```python
from build123d import *

# Parameters (mm, degrees)
BOSS_EXTRUDE1_DEPTH = 6
SKETCH2_W           = 7.6
SKETCH2_H           = 8.4
BOSS_EXTRUDE2_DEPTH = 4
SKETCH3_W           = 40
SKETCH3_H           = 30
BOSS_EXTRUDE3_DEPTH = 6
BOSS_EXTRUDE4_DEPTH = 2.5
BOSS_EXTRUDE5_DEPTH = 2.5
FILLET1_R           = 10
SKETCH8_R           = 1.6
CUT_EXTRUDE1_DEPTH  = 34.2
FILLET3_R           = 0.5
FILLET4_R           = 0.5
FILLET5_R           = 0.5
SKETCH9_R           = 14.329528823
CUT_EXTRUDE2_DEPTH  = 12.2
CUT_EXTRUDE3_DEPTH  = 3
FILLET6_R           = 0.5
FILLET7_R           = 1
FILLET8_R           = 1.5
FILLET9_R           = 0.3


with BuildPart() as part:
    # Sketch1 → Boss-Extrude1 (new body, symmetric)
    with BuildSketch(Plane(origin=(0, 0, 0), x_dir=(1, 0, 0), z_dir=(0, 1, 0))):
        Polygon((-8, 0), (8, 0), (8, 3.6), (4.3, 7.2), (-4.3, 7.2), (-8, 3.6), align=None)
    extrude(amount=BOSS_EXTRUDE1_DEPTH, both=True)

    # Sketch2 → Boss-Extrude2 (add)
    with BuildSketch(Plane(origin=(0, 0, -7.2), x_dir=(-1, 0, 0), z_dir=(0, 0, -1))):
        Rectangle(SKETCH2_W, SKETCH2_H)
    extrude(amount=BOSS_EXTRUDE2_DEPTH)

    # Sketch3 → Boss-Extrude3 (add)
    with BuildSketch(Plane(origin=(0, 0, -11.2), x_dir=(-1, 0, 0), z_dir=(0, 0, -1))):
        Rectangle(SKETCH3_W, SKETCH3_H)
    extrude(amount=BOSS_EXTRUDE3_DEPTH)

    # Sketch6 → Boss-Extrude4 (add, symmetric)
    with BuildSketch(Plane.ZY.offset(10)):
        Polygon((-29.2, 8), (-17.2, 8), (-17.2, 12), (-33.2, 12), (-33.2, -12), (-25.2, -12), (-25.2, -8), (-29.2, -8), align=None)
    extrude(amount=BOSS_EXTRUDE4_DEPTH, both=True)

    # Sketch7 → Boss-Extrude5 (add, symmetric)
    with BuildSketch(Plane(origin=(10, 0, 0), x_dir=(0, 0, -1), z_dir=(1, 0, 0))):
        Polygon((25.2, 12), (25.2, 8), (29.2, 8), (29.2, -8), (17.2, -8), (17.2, -12), (33.2, -12), (33.2, 12), align=None)
    extrude(amount=BOSS_EXTRUDE5_DEPTH, both=True)

    # Fillet1
    fillet1_edges = [part.edges().sort_by_distance(p)[0] for p in [
        (-20, -15, -14.2),
        (-20, 15, -14.2),
        (20, 15, -14.2),
        (20, -15, -14.2),
    ]]
    fillet(fillet1_edges, radius=FILLET1_R)

    # Sketch8 → Cut-Extrude1 (cut, through all)
    with BuildSketch(Plane.XY):
        Circle(SKETCH8_R)
    extrude(amount=-CUT_EXTRUDE1_DEPTH, mode=Mode.SUBTRACT)

    # Fillet3
    fillet3_edges = [part.edges().sort_by_distance(p)[0] for p in [
        (-6.15, 6, -5.4),
        (-8, 6, -1.8),
        (0, 6, 0),
        (8, 6, -1.8),
        (6.15, 6, -5.4),
        (8, -6, -1.8),
        (0, -6, 0),
        (-8, -6, -1.8),
        (-6.15, -6, -5.4),
        (0, -6, -7.2),
        (6.15, -6, -5.4),
        (0, 6, -7.2),
    ]]
    fillet(fillet3_edges, radius=FILLET3_R)

    # Fillet4
    fillet4_edges = [part.edges().sort_by_distance(p)[0] for p in [
        (-20, 0, -11.2),
        (-20, 0, -17.2),
        (0, -15, -11.2),
        (20, 0, -11.2),
        (0, 15, -11.2),
        (17.071067812, 12.071067812, -11.2),
        (17.071067812, -12.071067812, -11.2),
        (-17.071067812, 12.071067812, -11.2),
        (-17.071067812, -12.071067812, -11.2),
        (0, -15, -17.2),
        (0, 15, -17.2),
        (20, 0, -17.2),
        (17.071067812, 12.071067812, -17.2),
        (17.071067812, -12.071067812, -17.2),
        (-17.071067812, 12.071067812, -17.2),
        (-17.071067812, -12.071067812, -17.2),
    ]]
    fillet(fillet4_edges, radius=FILLET4_R)

    # Fillet5
    fillet5_edges = [part.edges().sort_by_distance(p)[0] for p in [
        (-3.8, 0, -11.2),
        (0, 4.2, -11.2),
        (3.8, 0, -11.2),
        (0, -4.2, -11.2),
    ]]
    fillet(fillet5_edges, radius=FILLET5_R)

    # Sketch9 → Cut-Extrude2 (cut, through all)
    with BuildSketch(Plane.XY.offset(-11.2)):
        Circle(SKETCH9_R)
    extrude(amount=CUT_EXTRUDE2_DEPTH, mode=Mode.SUBTRACT)

    # Sketch10 → Cut-Extrude3 (cut)
    with BuildSketch(Plane.XY.offset(-11.2)):
        Polygon((3.5, 0), (1.75, 3.031088913), (-1.75, 3.031088913), (-3.5, 0), (-1.75, -3.031088913), (1.75, -3.031088913), align=None)
    extrude(amount=-CUT_EXTRUDE3_DEPTH, mode=Mode.SUBTRACT)

    # Fillet6
    fillet6_edges = [part.edges().sort_by_distance(p)[0] for p in [
        (2.625, -1.515544457, -11.2),
        (2.625, 1.515544457, -11.2),
        (0, 3.031088913, -11.2),
        (-2.625, 1.515544457, -11.2),
        (-2.625, -1.515544457, -11.2),
        (0, -3.031088913, -11.2),
    ]]
    fillet(fillet6_edges, radius=FILLET6_R)

    # Fillet7
    fillet7_edges = [part.edges().sort_by_distance(p)[0] for p in [
        (-10, 8, -29.2),
        (-10, 12, -33.2),
        (-10, -12, -33.2),
        (-10, -12, -25.2),
        (-10, -8, -25.2),
        (-10, -8, -29.2),
        (10, -12, -33.2),
        (10, 12, -33.2),
        (10, 12, -25.2),
        (10, 8, -25.2),
        (10, 8, -29.2),
        (10, -8, -29.2),
    ]]
    fillet(fillet7_edges, radius=FILLET7_R)

    # Fillet8
    fillet8_edges = [part.edges().sort_by_distance(p)[0] for p in [
        (-7.5, 10, -17.2),
        (-10, 8, -17.2),
        (-10, 12, -17.2),
        (-12.5, 10, -17.2),
        (10, -12, -17.2),
        (7.5, -10, -17.2),
        (10, -8, -17.2),
        (12.5, -10, -17.2),
    ]]
    fillet(fillet8_edges, radius=FILLET8_R)

    # Fillet9
    fillet9_edges = [part.edges().sort_by_distance(p)[0] for p in [
        (-1.6, 0, -17.2),
    ]]
    fillet(fillet9_edges, radius=FILLET9_R)


solid = part.part
```
The listing builds one solid part. Answer for the finished solid, in the listing's coordinates (mm). A direction names the side the tool comes from. Coordinates: 2 decimals unless noted, no trailing zeros. Loops run counter-clockwise (first coordinate to the right, second up) from the corner with the lowest first, then second, coordinate; pieces in that order, holes last. Notation, with made-up numbers: M 37,-10 L 50,-10 A17 cw 50,18 Z; hole C 54.25,17.25 d11. An arc over 180 degrees is marked long. Answer as a JSON object with one key per item and string values. Group by question number.
Item 1: Each of these flat-tipped pins is pushed along its axis until it touches: P1, Ø2.5, axis at x = -10, z = -23.5, coming from the +Y side; P2, Ø11.5, axis at y = -2, z = -28.5, coming from the -X side; P3, Ø4, axis at x = 0, y = 0, coming from the +Z side. Where does it stop, or does it pass through?
Item 2: Which of the six approach directions +Z, -Z, +X, -X, +Y, -Y give full straight-line access (tool end or side, diameter ignored) to faces 1 (the face through (-10, -12, -29)), 2 (the face through (10.035, 8.301, -25.485)), 3 (the face through (-10.035, -11.715, -25.501)), 4 (the face through (10, -8, -24)), 5 (the face through (2.64, 1.49, -12.93))?
Item 3: Determine the mould class of faces 6 (the face through (-9.965, -8.301, -25.485)), 7 (the face through (-6.847, 10.049, -17.462)), 8 (the face through (7.5, 0, -31)) for opening direction X: +X half, -X half, draft (parallel to the pull), parting line (faces both ways), or undercut.
Item 4: Section A-A (z = -12.5) is taken. Write down the section's boundary in (x, y).
Item 5: Section D-D (z = -19.5) is taken. Write down the section's boundary in (x, y).
Item 6: Section C-C (z = -27.25) is taken. Write down the section's boundary in (x, y).
Item 7: Section B-B (x = 0) is taken. Write down the section's boundary in (y, z).
Item 8: Consider L1, parallel to Z at x = -11.5, y = -10; L2, parallel to Y at x = 0, z = -14.95; L3, parallel to X at y = 7, z = -31.5. Determine where each line is inside the solid, lowest interval first.
Solved:
{
 "1": {"P1": "stops at y = 12", "P2": "stops at x = -12.5", "P3": "stops at z = -14.2"},
 "2": {"face 1": "-Z, +X, -X, -Y", "face 2": "+X", "face 3": "-X, -Y", "face 4": "+X, -X", "face 5": "+Z"},
 "3": {"face 6": "draft", "face 7": "+X half", "face 8": "undercut"},
 "4": {"outline": "M -20,-5 A10 ccw -10,-15 L 10,-15 A10 ccw 20,-5 L 20,5 A10 ccw 10,15 L -10,15 A10 ccw -20,5 Z; hole M -3.5,0 L -1.75,-3.03 L 1.75,-3.03 L 3.5,0 L 1.75,3.03 L -1.75,3.03 Z"},
 "5": {"outline": "M -12.5,8 L -7.5,8 L -7.5,12 L -12.5,12 Z; M 7.5,-12 L 12.5,-12 L 12.5,-8 L 7.5,-8 Z"},
 "6": {"outline": "M -12.5,-12 L -7.5,-12 L -7.5,-8 L -12.5,-8 Z; M -12.5,8 L -7.5,8 L -7.5,12 L -12.5,12 Z; M 7.5,-12 L 12.5,-12 L 12.5,-8 L 7.5,-8 Z; M 7.5,8 L 12.5,8 L 12.5,12 L 7.5,12 Z"},
 "7": {"outline": "M -15,-16.7 A0.5 ccw -14.5,-17.2 L -1.9,-17.2 A0.3 ccw -1.6,-16.9 L -1.6,-14.2 L -3.03,-14.2 L -3.03,-11.7 A0.5 ccw -3.53,-11.2 L -14.5,-11.2 A0.5 ccw -15,-11.7 Z; M 1.6,-16.9 A0.3 ccw 1.9,-17.2 L 14.5,-17.2 A0.5 ccw 15,-16.7 L 15,-11.7 A0.5 ccw 14.5,-11.2 L 3.53,-11.2 A0.5 ccw 3.03,-11.7 L 3.03,-14.2 L 1.6,-14.2 Z"},
 "8": {"L1": "z = -33.2 to -25.2, -17.2 to -11.2", "L2": "y = -15 to -1.6, 1.6 to 15", "L3": "x = -12.5 to -7.5, 7.5 to 12.5"}
}
